```python
from build123d import *

# Parameters (mm, degrees)
SKETCH2_R           = 1.5
BOSS_EXTRUDE1_DEPTH = 1.5
SKETCH3_W           = 10.6
SKETCH3_H           = 15.6
BOSS_EXTRUDE2_DEPTH = 1.5


with BuildPart() as part:
    # Sketch2 → Boss-Extrude1 (new body)
    with BuildSketch(Plane(origin=(0, 0, 0), x_dir=(1, 0, 0), z_dir=(0, 1, 0))):
        with BuildLine():
            Line((15, 18), (15, 2))
            Line((15, 2), (20, 2))
            Line((20, 2), (20, 0))
            Line((20, 0), (15, 0))
            Line((15, 0), (0, 0))
            Line((0, 0), (0, 6.5))
            Line((0, 6.5), (-2, 6.5))
            ThreePointArc((-2, 6.5), (-5.5, 10), (-2, 13.5))
            Line((-2, 13.5), (0, 13.5))
            Line((0, 13.5), (0, 20))
            Line((0, 20), (15, 20))
            Line((15, 20), (20, 20))
            Line((20, 20), (20, 18))
            Line((20, 18), (15, 18))
        make_face()
        with Locations(Location((-2, 10, 0), (0, 0, 270))):
            Circle(SKETCH2_R, mode=Mode.SUBTRACT)
    extrude(amount=BOSS_EXTRUDE1_DEPTH)

    # Sketch3 → Boss-Extrude2 (add)
    with BuildSketch(Plane.XZ):
        with Locations((7.5, -10)):
            Rectangle(SKETCH3_W, SKETCH3_H)
    extrude(amount=BOSS_EXTRUDE2_DEPTH)


solid = part.part
```
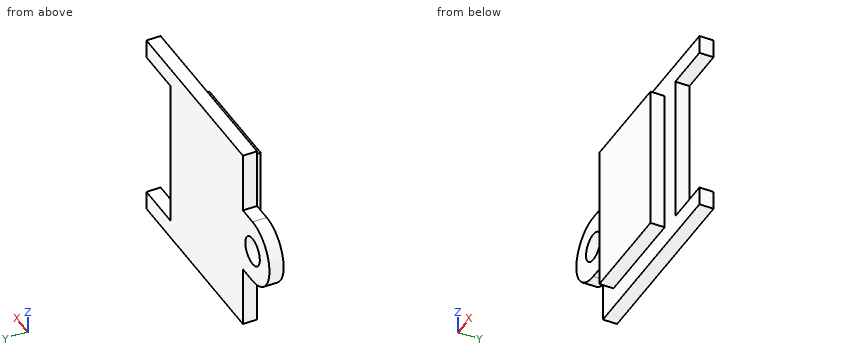
For this review, take the finished solid that the model builds, in its own axes (mm). Round coordinates to 2 decimals unless told otherwise and drop trailing zeros. Write each loop counter-clockwise with the first axis right and the second up, starting at its lowest first coordinate (ties: lowest second). Pieces come first, ordered by that corner, then holes. Notation, with made-up numbers: (-6.75, 18.5) -> (-0.75, 18.5) arc R18 cw to (-0.75, 44.5) -> close; hole circle Ø11 at (-28.75, 82.25). An arc over 180 degrees is marked (long way). Use one line per item in the form item = value.
Q1. Consider section B-B (x = 17.5). State the section outline as (y, z) points.
Resolved:
outline = (0, -20) -> (1.5, -20) -> (1.5, -18) -> (0, -18) -> close; (0, -2) -> (1.5, -2) -> (1.5, 0) -> (0, 0) -> close
Q2. Consider section D-D (x = 8). State the section outline as (y, z) points, then the cut area to 3 significant figures.
Resolved:
outline = (-1.5, -17.8) -> (0, -17.8) -> (0, -20) -> (1.5, -20) -> (1.5, 0) -> (0, 0) -> (0, -2.2) -> (-1.5, -2.2) -> close
area = 53.4 mm²
Q3. Consider section A-A (z = -10). State the section outline as (x, y) points, then the cut area to 4 significant figures.
Resolved:
outline = (-5.5, 0) -> (-3.5, 0) -> (-3.5, 1.5) -> (-5.5, 1.5) -> close; (-0.5, 0) -> (2.2, 0) -> (2.2, -1.5) -> (12.8, -1.5) -> (12.8, 0) -> (15, 0) -> (15, 1.5) -> (-0.5, 1.5) -> close
area = 42.15 mm²
Q4. Clearance check with flat-ended pins moving along their axes: pin 1 Ø0.8 at (y, z) = (-1, -12) entering from +X; pin 2 Ø1.6 at (y, z) = (0.5, -16) entering from -X; pin 3 Ø1.2 at (y, z) = (-1, -13.5) entering from -X. State where each tip first meets the part, or that it passes through.
Resolved:
pin_1 = 12.8
pin_2 = 0
pin_3 = 2.2
Q5. Consider section C-C (y = 0.8). State the section outline as (x, z) points.
Resolved:
outline = (-2, -13.5) -> (0, -13.5) -> (0, -20) -> (20, -20) -> (20, -18) -> (15, -18) -> (15, -2) -> (20, -2) -> (20, 0) -> (0, 0) -> (0, -6.5) -> (-2, -6.5) arc R3.5 ccw to start; hole circle Ø3 at (-2, -10)
Q6. To check wall thickness, follow probe 1 along Z at (x, y) = (17.5, 1); probe 2 along X at (y, z) = (0.5, -10); probe 3 along X at (y, z) = (-0.65, -12.25). State the ranges of each line that lie inside material, in increasing order. Write a range as from..to.
Resolved:
probe_1 = -20..-18, -2..0
probe_2 = -5.5..-3.5, -0.5..15
probe_3 = 2.2..12.8
